```python
from build123d import *

# Parameters (mm, degrees)
SKETCH1_W           = 206
SKETCH1_H           = 66
SKETCH1_R           = 2
SKETCH1_R_2         = 11
SKETCH1_W_2         = 5
SKETCH1_H_2         = 5
SKETCH1_H_3         = 4
BOSS_EXTRUDE4_DEPTH = 5
FILLET9_R           = 5


with BuildPart() as part:
    # Sketch1 → Boss-Extrude4 (new body)
    with BuildSketch(Plane(origin=(0, 0, 0), x_dir=(1, 0, 0), z_dir=(0, 1, 0))):
        with Locations((5.102707087, 13.156325227)):
            Rectangle(SKETCH1_W, SKETCH1_H)
        with Locations(Location((-54.897292913, 40.656325227, 0), (0, 0, 270))):
            Circle(SKETCH1_R, mode=Mode.SUBTRACT)
        with Locations(Location((-54.897292913, -14.343674773, 0), (0, 0, 90))):
            Circle(SKETCH1_R, mode=Mode.SUBTRACT)
        with Locations(Location((65.102707087, -14.343674773, 0), (0, 0, 270))):
            Circle(SKETCH1_R, mode=Mode.SUBTRACT)
        with Locations(Location((65.102707087, 40.656325227, 0), (0, 0, 90))):
            Circle(SKETCH1_R, mode=Mode.SUBTRACT)
        with Locations(Location((-74.397292913, 13.156325227, 0), (0, 0, 270))):
            Circle(SKETCH1_R_2, mode=Mode.SUBTRACT)
        with Locations(Location((-46.397292913, 13.156325227, 0), (0, 0, 270))):
            Circle(SKETCH1_R, mode=Mode.SUBTRACT)
        with Locations(Location((56.602707087, 13.156325227, 0), (0, 0, 90))):
            Circle(SKETCH1_R, mode=Mode.SUBTRACT)
        with Locations((57.602707087, 40.656325227)):
            Rectangle(SKETCH1_W_2, SKETCH1_H_2, mode=Mode.SUBTRACT)
        with Locations((-62.397292913, 40.656325227)):
            Rectangle(SKETCH1_W_2, SKETCH1_H_2, mode=Mode.SUBTRACT)
        with Locations((-47.397292913, 40.656325227)):
            Rectangle(SKETCH1_W_2, SKETCH1_H_2, mode=Mode.SUBTRACT)
        with Locations((72.602707087, 40.656325227)):
            Rectangle(SKETCH1_W_2, SKETCH1_H_2, mode=Mode.SUBTRACT)
        with Locations((72.602707087, -14.343674773)):
            Rectangle(SKETCH1_W_2, SKETCH1_H_2, mode=Mode.SUBTRACT)
        with Locations((57.602707087, -14.343674773)):
            Rectangle(SKETCH1_W_2, SKETCH1_H_2, mode=Mode.SUBTRACT)
        with Locations((-47.397292913, -14.343674773)):
            Rectangle(SKETCH1_W_2, SKETCH1_H_2, mode=Mode.SUBTRACT)
        with Locations((-62.397292913, -14.343674773)):
            Rectangle(SKETCH1_W_2, SKETCH1_H_2, mode=Mode.SUBTRACT)
        with Locations((-46.397292913, 20.156325227)):
            Rectangle(SKETCH1_W_2, SKETCH1_H_3, mode=Mode.SUBTRACT)
        with Locations((-46.397292913, 6.156325227)):
            Rectangle(SKETCH1_W_2, SKETCH1_H_3, mode=Mode.SUBTRACT)
        with Locations((56.602707087, 6.156325227)):
            Rectangle(SKETCH1_W_2, SKETCH1_H_3, mode=Mode.SUBTRACT)
        with Locations((56.602707087, 20.156325227)):
            Rectangle(SKETCH1_W_2, SKETCH1_H_3, mode=Mode.SUBTRACT)
        Polygon((6.068183228, 4.156325227), (53.102707087, 4.156325227), (53.102707087, 22.156325227), (6.068183228, 22.156325227), (6.102707086, 27.656216871), (-8.397292913, 27.656325227), (-8.397292913, 22.156325227), (-42.897292913, 22.156325227), (-42.897292913, 4.156325227), (-8.397292913, 4.156325227), align=None, mode=Mode.SUBTRACT)
    extrude(amount=BOSS_EXTRUDE4_DEPTH)

    # Fillet9
    fillet9_edges = [part.edges().sort_by_distance(p)[0] for p in [
        (-97.897292913, 2.5, -46.156325227),
        (108.102707087, 2.5, -46.156325227),
        (108.102707087, 2.5, 19.843674773),
        (-97.897292913, 2.5, 19.843674773),
    ]]
    fillet(fillet9_edges, radius=FILLET9_R)


solid = part.part
```
Source: CAD feature listing. Evaluate the final solid. Frame: model axes, mm. Coordinates: 2 decimals unless noted, no trailing zeros. Loops run counter-clockwise (first coordinate to the right, second up) from the corner with the lowest first, then second, coordinate; pieces in that order, holes last. Notation, with made-up numbers: M -27.75,13.5 L 24.25,13.5 A14 cw 24.25,27.5 Z; hole C 70.5,14.5 d4. An arc over 180 degrees is marked long. Put each result on its own line as item: value. Start each with the question number.
1) Contact query for a flat-ended pin moving along its axis: pin 1 Ø3 at (x, z) = (65.1, -40.66) entering from -Y. Output: stop coordinate, or through.
2) Cut plane A-A on x = 12. Return the cut outline in (y, z), then the cut area to 3 significant figures.
3) Cut plane B-B on x = -81. Return the cut outline in (y, z).
4) Cut plane C-C on y = 3.9. Give the number of separate pieces and of enclosed holes in the cut face, then the cut area to 3 significant figures.
5) Ray query, L1, parallel to X at y = 3, z = -13; L2, parallel to Z at x = -62, y = 3.2; L3, parallel to X at y = 3.7, z = -24.5. Return the intervals inside material, ascending. Write a range as from..to.
6) Pull-direction query (Z, two-part tool) for faces 1 (the face through (4, 2, 19.844)), 2 (the face through (4, 2, -46.156)), 3 (the face through (73, 2, 11.844)); classes: pulls with the +Z half, pulls with the -Z half, needs draft (parallel to the pull), parting line crosses it, or undercut.
The answers:
1. pin 1: passes through
2. outline: M 0,-46.16 L 5,-46.16 L 5,-22.16 L 0,-22.16 Z; M 0,-4.16 L 5,-4.16 L 5,19.84 L 0,19.84 Z
2. area: 240 mm²
3. outline: M 0,-46.16 L 5,-46.16 L 5,-21.95 L 0,-21.95 Z; M 0,-4.36 L 5,-4.36 L 5,19.84 L 0,19.84 Z
4. separate pieces: 1
4. enclosed holes: 20
4. area: 11,000 mm²
5. L1: x = -97.9..-85.4, -63.4..-48.39, -44.4..-42.9, 53.1..54.61, 58.6..108.1
5. L2: z = -46.16..-43.16, -38.16..11.84, 16.84..19.84
5. L3: x = -97.9..-8.4, 6.08..108.1
6. face 1: pulls with the +Z half
6. face 2: pulls with the -Z half
6. face 3: undercut
